from build123d import *

# Parameters (mm, degrees)
BOSS_EXTRUDE1_START = -54
SKETCH1_R           = 65
BOSS_EXTRUDE1_DEPTH = 12
SKETCH2_R           = 54.25
CUT_EXTRUDE1_DEPTH  = 6
SKETCH3_R           = 50.25
CUT_EXTRUDE2_DEPTH  = 93.119487623
SKETCH4_R           = 62.5
CUT_EXTRUDE3_DEPTH  = 2.16
BOSS_EXTRUDE2_REACH = 139.31
SKETCH8_R           = 54.25
SKETCH8_R_2         = 50.25


# Read off the part's stored shape, not the designer's step: Cut-Revolve1
with BuildPart() as part:
    # Sketch1 → Boss-Extrude1 (new body)
    with BuildSketch(Plane(origin=(0, 0, 0), x_dir=(1, 0, 0), z_dir=(0, 1, 0)).offset(BOSS_EXTRUDE1_START)):
        with Locations(Location((0, 0, 0), (0, 0, 270))):
            Circle(SKETCH1_R)
    extrude(amount=BOSS_EXTRUDE1_DEPTH)

    # Sketch2 → Cut-Extrude1 (cut)
    with BuildSketch(Plane(origin=(0, -42, 0), x_dir=(1, 0, 0), z_dir=(0, 1, 0))):
        with Locations(Location((0, 0, 0), (0, 0, 270))):
            Circle(SKETCH2_R)
    extrude(amount=-CUT_EXTRUDE1_DEPTH, mode=Mode.SUBTRACT)

    # Sketch3 → Cut-Extrude2 (cut, through all)
    with BuildSketch(Plane(origin=(0, -48, 0), x_dir=(1, 0, 0), z_dir=(0, 1, 0))):
        with Locations(Location((0, 0, 0), (0, 0, 270))):
            Circle(SKETCH3_R)
    extrude(amount=-CUT_EXTRUDE2_DEPTH, mode=Mode.SUBTRACT)

    # Sketch4 → Cut-Extrude3 (cut)
    with BuildSketch(Plane(origin=(0, -42, 0), x_dir=(1, 0, 0), z_dir=(0, 1, 0))):
        with Locations(Location((0, 0, 0), (0, 0, 270))):
            Circle(SKETCH4_R)
    extrude(amount=-CUT_EXTRUDE3_DEPTH, mode=Mode.SUBTRACT)

    # Cut-Revolve1 outline → Cut-Revolve1 (revolve, cut)
    with BuildSketch(Plane.XY):
        with BuildLine():
            Line((65, -50.575), (65, -47.425))
            ThreePointArc((65, -47.425), (63.841807889, -49), (65, -50.575))
        make_face()
    revolve(axis=Axis((0, 0, 0), (0, 1, 0)), mode=Mode.SUBTRACT)


with BuildPart() as body_2:
    # Mirror5: mirrored copy
    add(part.part.mirror(Plane.ZX))

    # Sketch8 → Boss-Extrude2 (add, up to next)
    with BuildSketch(Plane(origin=(0, -48, 0), x_dir=(1, 0, 0), z_dir=(0, 1, 0)), mode=Mode.PRIVATE) as boss_extrude2_sk1:
        with Locations(Location((0, 0, 0), (0, 0, 270))):
            Circle(SKETCH8_R)
        with Locations(Location((0, 0, 0), (0, 0, 270))):
            Circle(SKETCH8_R_2, mode=Mode.SUBTRACT)
    boss_extrude2_tool1 = extrude(boss_extrude2_sk1.sketch, amount=BOSS_EXTRUDE2_REACH, mode=Mode.PRIVATE) - body_2.part

    add(part.part)  # Boss-Extrude2 merges part
    add(boss_extrude2_tool1.solids().sort_by_distance((0, -48, -52.715578))[0])


solid = body_2.part
Read the model definition and answer for the solid it produces. Units are mm, in the model's axes. A direction names the side the tool comes from. Coordinates: 2 decimals unless noted, no trailing zeros. Loops run counter-clockwise (first coordinate to the right, second up) from the corner with the lowest first, then second, coordinate; pieces in that order, holes last.
Q1. The part is cut by section C-C on y = 36. Write down the section's boundary in (x, z).
Q2. Which of the six approach directions +Z, -Z, +X, -X, +Y, -Y give full straight-line access (tool end or side, diameter ignored) to faces 5 (the face through (19.52, -44.75, 62)), 6 (the face through (51, -44.16, -19))?
Q3. Consider probe 1 along X at (y, z) = (-42.55, 0); probe 2 along Y at (x, z) = (5.5, -56); probe 3 along Z at (x, y) = (44, -39). Determine where each line is inside the solid, lowest interval first.
Q4. Each of these flat-tipped pins is pushed along its axis until it touches: pin 1 Ø2 at (x, y) = (5, 33.5) entering from +Z; pin 2 Ø6 at (x, y) = (-15.5, 10) entering from -Z; pin 3 Ø12 at (y, z) = (-12, -0.5) entering from +X. Where does it stop, or does it pass through?
Q5. The mould has two halves that part along X. Classify faces 1 (the face through (2.2, 0.8, -50.2)), 2 (the face through (-38.2, 54, 33.4)), 3 (the face through (19.52, -52.31, 62)), 4 (the face through (2.75, -43.06, -62.44)): +X half, -X half, draft (parallel to the pull), parting line (faces both ways), or undercut.
Results below:
1. outline: circle Ø108.5 at (0, 0); hole circle Ø100.5 at (0, 0)
2. face 5: +Y, -Y
2. face 6: none
3. probe 1: x = -65 to -62.5, -54.25 to -50.25, 50.25 to 54.25, 62.5 to 65
3. probe 2: y = -54 to -44.16, 44.16 to 54
3. probe 3: z = -31.73 to -24.27, 24.27 to 31.73
4. pin 1: stops at z = 54.1
4. pin 2: stops at z = -52.79
4. pin 3: stops at x = 54.25
5. face 1: undercut
5. face 2: draft
5. face 3: parting line
5. face 4: undercut
